Verification items for the finished model (mm, model axes). Face numbers are marked on the shaded views. A direction names the side the tool comes from. Give positions to 0.01 mm unless a question says otherwise; leave off trailing zeros. Order: outer loops, then holes, each group sorted by start corner. A loop starts at its lowest first (then second) coordinate and runs counter-clockwise, first axis right, second up. Notation, with made-up numbers: (27.25, 85) - (45.25, 85) arc R24 ccw to (45.25, 109) - close; hole circle Ø7 at (15, -36.75). An arc over 180 degrees is marked (long way). Answer as a JSON object with one key per item and string values.
```python
from build123d import *

# Parameters (mm, degrees)
F0_R          = 14.351
F1_DEPTH      = 12.7
F0_R_2        = 4.7625
F2_DEPTH      = 25.4
F2_DEPTH_BACK = 25.4
F3_DEPTH      = 12.7
F3_DEPTH_BACK = 12.7


with BuildPart() as f1:
    # F0 (on Top) → F1 (new body)
    with BuildSketch(Plane.XY):
        Polygon((-44.196002, -24.281906), (-44.196002, -49.681906), (32.003998, -49.681906), (32.003998, -24.281906), (46.278798, -24.281906), (46.278798, -11.581906), (-58.496202, -11.581906), (-58.496202, -24.281906), align=None)
        with Locations((-25.152352, -30.631906)):
            Circle(F0_R, mode=Mode.SUBTRACT)
        with Locations((12.947648, -30.631906)):
            Circle(F0_R, mode=Mode.SUBTRACT)
    extrude(amount=F1_DEPTH)

    # F0 (on Top) → F2 (join, two sides)
    with BuildSketch(Plane.XY) as f2_sk:
        with Locations((-25.152352, -30.631906)):
            Circle(F0_R)
        with Locations((-25.152352, -30.631906)):
            Circle(F0_R_2, mode=Mode.SUBTRACT)
        with Locations((12.947648, -30.631906)):
            Circle(F0_R)
        with Locations((12.947648, -30.631906)):
            Circle(F0_R_2, mode=Mode.SUBTRACT)
    extrude(amount=F2_DEPTH)
    extrude(f2_sk.sketch, amount=-F2_DEPTH_BACK)

    # F0 (on Top) → F3 (join, two sides)
    with BuildSketch(Plane.XY) as f3_sk:
        with Locations((-25.152352, -30.631906)):
            Circle(F0_R_2)
        with Locations((12.947648, -30.631906)):
            Circle(F0_R_2)
    extrude(amount=F3_DEPTH)
    extrude(f3_sk.sketch, amount=-F3_DEPTH_BACK)


solid = f1.part
```
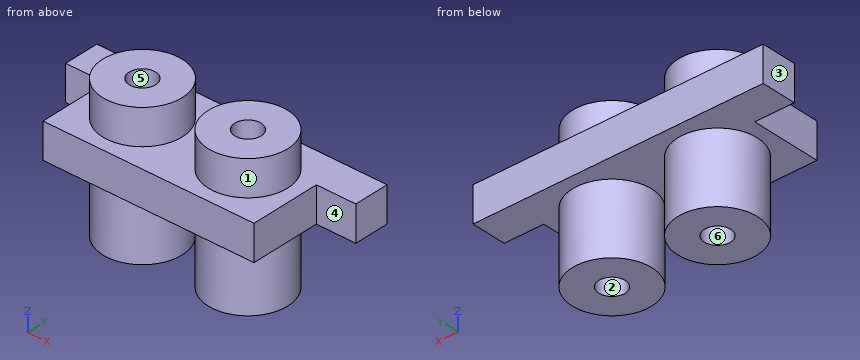
(1) Section check B-B (x = -34.5). Record the cut outline in (y, z), then the cut area to 3 significant figures.
Computed values:
{"outline": "(-49.68, 0) - (-41.52, 0) - (-41.52, -25.4) - (-19.74, -25.4) - (-19.74, 0) - (-11.58, 0) - (-11.58, 12.7) - (-19.74, 12.7) - (-19.74, 25.4) - (-41.52, 25.4) - (-41.52, 12.7) - (-49.68, 12.7) - close", "area": "1,310 mm²"}
(2) Release check for a two-part mould opening along Y. For the marked faces 1, 2 and 3 record: pulls with the +Y half, pulls with the -Y half, needs draft (parallel to the pull), parting line crosses it, or undercut.
Computed values:
{"face 1": "parting line crosses it", "face 2": "undercut", "face 3": "needs draft"}
(3) Access from +Z, -Z, +X, -X, +Y, -Y to the whole of each face (thin tool, end or side, straight path). Record for the marked faces 4, 5 and 6.
Computed values:
{"face 4": "+Z, -Z, +X, -Y", "face 5": "+Z", "face 6": "-Z"}
(4) Section check D-D (z = -15). Record the cut outline in (x, y) (1 decimal).
Computed values:
{"outline": "circle Ø28.7 at (-25.2, -30.6); circle Ø28.7 at (12.9, -30.6); hole circle Ø9.5 at (-25.2, -30.6); hole circle Ø9.5 at (12.9, -30.6)"}
(5) Section check C-C (y = -20). Record the cut outline in (x, z), then the cut area to 3 significant figures.
Computed values:
{"outline": "(-58.5, 0) - (-34.79, 0) - (-34.79, -25.4) - (-15.51, -25.4) - (-15.51, 0) - (3.31, 0) - (3.31, -25.4) - (22.59, -25.4) - (22.59, 0) - (46.28, 0) - (46.28, 12.7) - (22.59, 12.7) - (22.59, 25.4) - (3.31, 25.4) - (3.31, 12.7) - (-15.51, 12.7) - (-15.51, 25.4) - (-34.79, 25.4) - (-34.79, 12.7) - (-58.5, 12.7) - close", "area": "2,800 mm²"}
(6) Section check A-A (z = 1.5). Record the cut outline in (x, y).
Computed values:
{"outline": "(-58.5, -24.28) - (-44.2, -24.28) - (-44.2, -49.68) - (32, -49.68) - (32, -24.28) - (46.28, -24.28) - (46.28, -11.58) - (-58.5, -11.58) - close"}
(7) Material ranges on line 1 along X through (y, z) = (-33.5, -20); line 2 along Z through (x, y) = (37, -14); line 3 along Y through (x, z) = (12.5, -7), recorded low to high. Write a range as [from, to].
Computed values:
{"line 1": "x = [-39.21, -28.95], [-21.35, -11.09], [-1.11, 9.15], [16.75, 27.01]", "line 2": "z = [0, 12.7]", "line 3": "y = [-44.98, -16.29]"}
(8) Gauge pin test, flat ends, axial feed: pin 1 Ø6.5 at (x, z) = (-51.5, 4) entering from -Y; pin 2 Ø5 at (x, y) = (-24, -30) entering from +Z; pin 3 Ø4 at (y, z) = (-40.5, 8.5) entering from +X; pin 4 Ø1.5 at (x, y) = (33.5, -37) entering from +Z. Record the tip position at first contact, or that the pin passes through.
Computed values:
{"pin 1": "stops at y = -24.28", "pin 2": "stops at z = 12.7", "pin 3": "stops at x = 32", "pin 4": "passes through"}
